Autodesk Inventor part; units mm, degrees
ref_plane "YZ Plane" through (0, 0, 0) normal (1, 0, 0) x (0, 1, 0)
ref_plane "XZ Plane" through (0, 0, 0) normal (0, 1, 0) x (-1, 0, 0)
ref_plane "XY Plane" through (0, 0, 0) normal (0, 0, 1) x (1, 0, 0)
sketch "Sketch1" plane through (0, 0, 0) normal (0, 0, 1) x (1, 0, 0)
  line L0 (0, 0) -> (38.1, 0)
  line L1 (38.1, 0) -> (38.1, 253.0348)
  arc A0 (38.1, 507.0348) -> (38.1, 253.0348) centre (666.75, 380.0348) ccw
  line L2 (38.1, 507.0348) -> (38.1, 608.6348)
  line L3 (38.1, 608.6348) -> (0, 608.6348)
  line L4 (0, 608.6348) -> (0, 0)
  circle A1 centre (31.75, 151.4348) radius 3.3655
  circle A2 centre (31.75, 34.671) radius 3.3655
  circle A3 centre (12.7, 12.7) radius 3.3655
  circle A4 centre (12.7, 342.9) radius 3.3655
  circle A5 centre (12.7, 595.9348) radius 3.3655
  circle A6 centre (31.75, 12.7) radius 3.3655
  circle A7 centre (31.75, 253.0348) radius 3.3655
  circle A8 centre (31.75, 507.0348) radius 3.3655
  circle A9 centre (31.75, 595.9348) radius 3.3655
  line L5 (0, 557.8348) -> (0, 608.6348)
  line L6 (0, 50.8) -> (0, 0)
  line L7 (12.7, 342.9) -> (0, 304.3174) construction
  line L8 (0, 317.5) -> (0, 368.3)
  line L9 (0, 129.921) -> (12.7, 129.921) construction
  circle A10 centre (12.7, 129.921) radius 3.3655
  circle A11 centre (12.7, 174.371) radius 3.3655
  line L10 (9.3413, 197.482) -> (9.3413, 204.213)
  line L11 (16.0611, 204.488) -> (16.0611, 197.3435)
  arc A12 (16.0611, 204.488) -> (9.3413, 204.213) centre (12.6956, 204.488) ccw
  arc A13 (9.3413, 197.482) -> (16.0611, 197.3435) centre (12.6974, 197.231) ccw
  circle A14 centre (12.7, 217.188) radius 3.3655
  line L12 (35.1155, 268.8247) -> (0, 268.8247)
  dimension "d0" = 38.1
  dimension "d2" = 101.6
  dimension "d4" = 457.2
  dimension "d5" = 101.6
  dimension "d6" = 666.75
  dimension "d7" = 641.35
  dimension "d9" = 116.7638
  dimension "d10" = 6.35
  dimension "d11" = 6.35
  dimension "d13" = 12.7
  dimension "d14" = 12.7
  dimension "d16" = 12.7
  dimension "d17" = 342.9
  dimension "d19" = 12.7
  dimension "d20" = 12.7
  dimension "d22" = 6.35
  dimension "d24" = 6.35
  dimension "d25" = 6.731
  dimension "d26" = 6.35
  dimension "hole" = 6.731
  dimension "d28" = 6.35
  dimension "d45" = 12.7
  dimension "d47" = 12.7
  dimension "d54" = 6.731
  dimension "d55" = 3.3655
  dimension "d56" = 3.3655
  dimension "d58" = 6.731
  dimension "d59" = 12.7
  dimension "d68" = 18.22
  dimension "d69" = 90
  dimension "d70" = 90
  dimension "d71" = 22.0389
  dimension "d72" = 28.7587
  dimension "d73" = 478.7138
  dimension "d74" = 6.35
  dimension "d75" = 6.35
  dimension "d76" = 595.9348
  dimension "d77" = 404.1468
  dimension "d78" = 411.2913
  dimension "d79" = 25.4
  dimension "d80" = 25.4
  dimension "d81" = 434.2638
  dimension "d82" = 50.8
  dimension "d83" = 240.3348
  dimension "d84" = 291.1348
  dimension "d85" = 557.8348
extrude "Plate4" add sketch "Sketch1" along normal blind 3.048
sketch "Sketch5" plane through (0, 0, 3.048) normal (0, 0, 1) x (1, 0, 0)
  line L0 (38.1, 0) -> (38.1, 253.0348)
  line L1 (0, 0) -> (38.1, 0)
  line L2 (38.1, 0) -> (38.1, 25.4)
  line L3 (38.1, 25.4) -> (0, 25.4)
  line L4 (0, 25.4) -> (0, 0)
  dimension "d96" = 25.4
extrude "Cut1" cut sketch "Sketch5" against normal blind 3.048
sketch "Sketch7" plane through (0, 25.4, 3.048) normal (-1, 0, 0) x (0, -1, 0)
  line L0 (-583.2348, 0) -> (0, 0)
  line L1 (0, 0) -> (0, 22.352)
  line L2 (0, 22.352) -> (-583.2348, 22.352)
  line L3 (-583.2348, 22.352) -> (-583.2348, 0)
edge flange "Flange3" height 25.4 angle 90 thickness 3.048 bend radius 3.048 thickness toward (-1, 0, 0) relief tear relief width 3.048 relief depth 1.524 edges at (0, 317.0174, 3.048) wall of the first edge with corners at (0, 608.6348, 3.048) (0, 25.4, 3.048) (0, 25.4, 25.4) (0, 608.6348, 25.4)
bend "Bend3"
corner "Corner3"
sketch "Sketch8" plane through (-3.048, 25.4, 25.4) normal (0, -1, 0) x (1, 0, 0)
  line L0 (0, 0) -> (41.148, 0)
  line L1 (41.148, 0) -> (41.148, -25.4)
  line L2 (41.148, -25.4) -> (0, -25.4)
  line L3 (0, -25.4) -> (0, 0)
  point P0 (3.048, -25.4)
sketch "Sketch9" plane through (-3.048, 608.6348, 25.4) normal (0, 1, 0) x (1, 0, 0)
  line L0 (41.148, 25.4) -> (0, 25.4)
  line L1 (0, 25.4) -> (0, 0)
  line L2 (0, 0) -> (41.148, 0)
  line L3 (41.148, 0) -> (41.148, 25.4)
  point P0 (3.048, 25.4)
extrude "Extrusion1" cut sketch "Sketch9" against normal blind 320.675
extrude "Extrusion2" cut sketch "Sketch8" against normal blind 209.9818
equation "\"d97\" = Thickness"
equation "\"d25\" = hole"
equation "\"d109\" = BendReliefWidth"
equation "\"d110\" = BendReliefDepth"
equation "\"d111\" = MinimumRemnant"
equation "\"d112\" = BendRadius"
equation "\"d115\" = BendRadius"
equation "\"d116\" = CornerReliefSize"
equation "\"d117\" = GapSize"
equation "\"d118\" = JacobiRadiusSize"
equation "\"BendRadius\" = Thickness"
equation "\"BendReliefWidth\" = Thickness"
equation "\"BendReliefDepth\" = 0.5 * Thickness"
equation "\"CornerReliefSize\" = 4 * Thickness"
equation "\"MinimumRemnant\" = 2 * Thickness"
equation "\"TransitionRadius\" = BendRadius"
equation "\"JacobiRadiusSize\" = BendRadius"
equation "\"GapSize\" = Thickness"
equation "\"d29\" = BendRadius"
equation "\"d32\" = BendRadius"
equation "\"d38\" = BendRadius"
equation "\"d60\" = BendRadius"
properties part number "Claw - Arm - Top (R) v2"
For this review, take the finished solid that the model builds, in its own axes (mm). A direction names the side the tool comes from. Round coordinates to 2 decimals unless told otherwise and drop trailing zeros. Write each loop counter-clockwise with the first axis right and the second up, starting at its lowest first coordinate (ties: lowest second). Pieces come first, ordered by that corner, then holes. Notation, with made-up numbers: (61, -28) -> (109, -28) arc R37 ccw to (109, 8) -> close; hole circle Ø6 at (18.5, 0). An arc over 180 degrees is marked (long way). Use CSV: the item, a comma, the result in double quotes.
(1) Consider section A-A, the plane y = 257. Give the boundary of the cut face in (x, z), plus the area to 3 significant figures.
Computed values:
outline,"(-3.05, 6.1) arc R6.1 ccw to (3.05, 0) -> (37.31, 0) -> (37.31, 3.05) -> (3.05, 3.05) arc R3.05 cw to (0, 6.1) -> (0, 25.4) -> (-3.05, 25.4) -> close"
area,"185 mm²"
(2) Draft analysis for pull direction X (two halves, no side actions). For faces 1 (the face through (10, 235.382, 2)), 2 (the face through (31.3, 249.7, 1.5)), 3 (the face through (-1.31, 261.303, 1.833)), state which applies: +X half, -X half, draft (parallel to the pull), parting line (faces both ways), or undercut.
Computed values:
face 1,"draft"
face 2,"undercut"
face 3,"-X half"
(3) Consider section D-D, the plane y = 244.5. Give the boundary of the cut face in (x, z), plus the area to 3 significant figures.
Computed values:
outline,"(-3.05, 6.1) arc R6.1 ccw to (3.05, 0) -> (38.1, 0) -> (38.1, 3.05) -> (3.05, 3.05) arc R3.05 cw to (0, 6.1) -> (0, 25.4) -> (-3.05, 25.4) -> close"
area,"188 mm²"
(4) Clearance check with a flat-ended pin moving along its axis: P1, Ø4, axis at y = 259.5, z = 19.5, coming from the +X side. State where the tip first meets the part, or that it passes through.
Computed values:
P1,"x = 0"
(5) For faces 4 (the face through (-2, 261, 25.4)), 5 (the face through (20, 262, 3.048)), list the 3-axis set-ups (+Z, -Z, +X, -X, +Y, -Y) from which the entire face can be reached by the end or side of a thin tool; tool diameter is ignored.
Computed values:
face 4,"+Z, +X, -X, +Y, -Y"
face 5,"+Z, +X, +Y, -Y"
(6) To check wall thickness, follow L1, parallel to Y at x = 31.75, z = 0.8; L2, parallel to X at y = 254, z = 8; L3, parallel to Z at x = 21, y = 265. State the ranges of each line that lie inside material, in increasing order. Write a range as [from, to].
Computed values:
L1,"[235.38, 249.67], [256.4, 287.96]"
L2,"[-3.05, 0]"
L3,"[0, 3.05]"
(7) Consider section B-B, the plane x = 17. Give the boundary of the cut face in (y, z).
Computed values:
outline,"(235.38, 0) -> (287.96, 0) -> (287.96, 3.05) -> (235.38, 3.05) -> close"
(8) Consider section C-C, the plane z = 20.5. Give the boundary of the cut face in (x, y), plus the area to 3 significant figures.
Computed values:
outline,"(-3.05, 235.38) -> (0, 235.38) -> (0, 287.96) -> (-3.05, 287.96) -> close"
area,"160 mm²"
